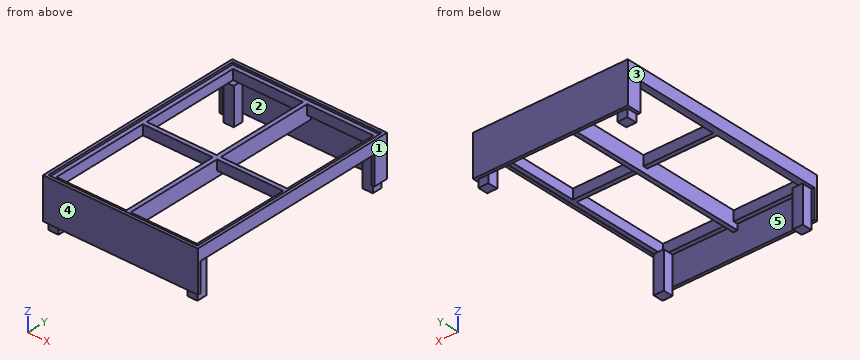
```python
from build123d import *

# Parameters (mm, degrees)
F0_W      = 1371.6
F0_H      = 1905
F0_W_2    = 1320.8
F0_H_2    = 1854.2
F1_DEPTH  = 365.125
F2_W      = 38.1
F2_H      = 139.7
F3_DEPTH  = 1854.2
F4_W      = 1854.2
F4_H      = 88.9
F5_DEPTH  = 38.1
F6_W      = 1854.2
F6_H      = 88.9
F7_DEPTH  = 38.1
F8_W      = 1752.6
F8_H      = 254
F9_DEPTH  = 1371.601
F10_DEPTH = 1752.6
F11_W     = 38.1
F11_H     = 88.9
F12_DEPTH = 1270
F13_W     = 38.1
F13_H     = 88.9
F14_DEPTH = 1270
F15_W     = 38.1
F15_H     = 88.9
F16_DEPTH = 1270
F17_W     = 88.9
F17_H     = 88.9
F18_DEPTH = 327.025
F19_W     = 88.9
F19_H     = 88.9
F20_DEPTH = 327.025
F21_W     = 88.9
F21_H     = 88.9
F22_DEPTH = 327.025
F23_W     = 88.9
F23_H     = 88.9
F24_DEPTH = 327.025


with BuildPart() as f1:
    # F0 (on Top) → F1 (new body)
    with BuildSketch(Plane.XY):
        Rectangle(F0_W, F0_H)
        Rectangle(F0_W_2, F0_H_2, mode=Mode.SUBTRACT)
    extrude(amount=F1_DEPTH)

    # F2 (on face) → F3 (join, through all)
    with BuildSketch(Plane.XZ.offset(-927.1)):
        with Locations((15.875, 276.225)):
            Rectangle(F2_W, F2_H)
    extrude(amount=F3_DEPTH)

    # F4 (on face) → F5 (join)
    with BuildSketch(Plane.YZ.offset(-660.4)):
        with Locations((0, 301.625)):
            Rectangle(F4_W, F4_H)
    extrude(amount=F5_DEPTH)

    # F6 (on face) → F7 (join)
    with BuildSketch(Plane(origin=(660.4, 0, 0), x_dir=(0, -1, 0), z_dir=(-1, 0, 0))):
        with Locations((0, 301.625)):
            Rectangle(F6_W, F6_H)
    extrude(amount=F7_DEPTH)

    # F8 (on face) → F9 (cut, through all)
    with BuildSketch(Plane.YZ.offset(685.8)):
        with Locations((-50.8, 127)):
            Rectangle(F8_W, F8_H)
    extrude(amount=-F9_DEPTH, mode=Mode.SUBTRACT)

    # F10 (add, through all): a face of the model
    f10_faces = [f1.faces().sort_by_distance(p)[0] for p in [
        (15.875, 825.5, 230.1875),
    ]]
    extrude(f10_faces, amount=F10_DEPTH)

    # F11 (on face) → F12 (join)
    with BuildSketch(Plane.YZ.offset(-622.3)):
        with Locations((908.05, 301.625)):
            Rectangle(F11_W, F11_H)
    extrude(amount=F12_DEPTH)

    # F13 (on face) → F14 (join)
    with BuildSketch(Plane.YZ.offset(-622.3)):
        with Locations((-908.05, 301.625)):
            Rectangle(F13_W, F13_H)
    extrude(amount=F14_DEPTH)

    # F15 (on face) → F16 (join)
    with BuildSketch(Plane.YZ.offset(-622.3)):
        with Locations((0, 301.625)):
            Rectangle(F15_W, F15_H)
    extrude(amount=F16_DEPTH)

    # F17 (on face) → F18 (join)
    with BuildSketch(Plane(origin=(0, 0, 257.175), x_dir=(1, 0, 0), z_dir=(0, 0, -1))):
        with Locations((-615.95, 882.65)):
            Rectangle(F17_W, F17_H)
    extrude(amount=F18_DEPTH)

    # F19 (on face) → F20 (join)
    with BuildSketch(Plane(origin=(0, 0, 257.175), x_dir=(1, 0, 0), z_dir=(0, 0, -1))):
        with Locations((615.95, 882.65)):
            Rectangle(F19_W, F19_H)
    extrude(amount=F20_DEPTH)

    # F21 (on face) → F22 (join)
    with BuildSketch(Plane(origin=(0, 0, 257.175), x_dir=(1, 0, 0), z_dir=(0, 0, -1))):
        with Locations((-615.95, -882.65)):
            Rectangle(F21_W, F21_H)
    extrude(amount=F22_DEPTH)

    # F23 (on face) → F24 (join)
    with BuildSketch(Plane(origin=(0, 0, 257.175), x_dir=(1, 0, 0), z_dir=(0, 0, -1))):
        with Locations((615.95, -882.65)):
            Rectangle(F23_W, F23_H)
    extrude(amount=F24_DEPTH)


solid = f1.part
```
Read the model definition and answer for the solid it produces. Units are mm, in the model's axes. Face numbers are marked on the shaded views. A direction names the side the tool comes from. Coordinates: 2 decimals unless noted, no trailing zeros. Order: outer loops, then holes, each group sorted by start corner. A loop starts at its lowest first (then second) coordinate and runs counter-clockwise, first axis right, second up. Notation, with made-up numbers: (-38, 52) - (13, 52) arc R18 cw to (13, 87) - close; hole circle Ø6 at (59, 25.5). An arc over 180 degrees is marked (long way). Answer as a JSON object with one key per item and string values. Group by question number.
Item 1: Consider probe 1 along Y at (x, z) = (-561.5, 299); probe 2 along X at (y, z) = (-777, 334) (3 decimals); probe 3 along Y at (x, z) = (-570.5, 108.5). Determine where each line is inside the solid, lowest interval first. Write a range as from..to.
Item 2: Section C-C (y = 122) is taken. Give the vertices of the cut face in (x, z) (3 decimals).
Item 3: Section B-B (x = 305.5) is taken. Give the vertices of the cut face in (y, z) (3 decimals).
Item 4: A flat-ended cylindrical pin translates along its axis: P1, Ø4, axis at x = 538.5, y = 9, coming from the +Z side (3 decimals). Find the tip coordinate at first contact, or state that the pin passes through.
Item 5: Section D-D (z = 290) is taken. Give the vertices of the cut face in (x, y) (3 decimals).
Item 6: Section A-A (z = 149) is taken. Give the vertices of the cut face in (x, y).
Item 7: A tool of negligible diameter and unlimited length cuts with its end or side. For the marked faces 1 and 2, from which of +Z, -Z, +X, -X, +Y, -Y can it reach the whole face along a straight path? Write none if from no direction.
Item 8: The mould has two halves that part along Y. Classify the marked faces 3, 4 and 5: +Y half, -Y half, draft (parallel to the pull), parting line (faces both ways), or undercut.
Results are:
{
 "1": {"probe 1": "y = -952.5..-889, -19.05..19.05, 889..952.5", "probe 2": "x = -685.8..-622.3, -3.175..34.925, 622.3..685.8", "probe 3": "y = -952.5..-927.1, 927.1..952.5"},
 "2": {"outline": "(-685.8, 254) - (-660.4, 254) - (-660.4, 257.175) - (-622.3, 257.175) - (-622.3, 346.075) - (-660.4, 346.075) - (-660.4, 365.125) - (-685.8, 365.125) - close; (-3.175, 206.375) - (34.925, 206.375) - (34.925, 346.075) - (-3.175, 346.075) - close; (622.3, 257.175) - (660.4, 257.175) - (660.4, 254) - (685.8, 254) - (685.8, 365.125) - (660.4, 365.125) - (660.4, 346.075) - (622.3, 346.075) - close"},
 "3": {"outline": "(-952.5, 0) - (-927.1, 0) - (-927.1, 257.175) - (-889, 257.175) - (-889, 346.075) - (-927.1, 346.075) - (-927.1, 365.125) - (-952.5, 365.125) - close; (-19.05, 257.175) - (19.05, 257.175) - (19.05, 346.075) - (-19.05, 346.075) - close; (889, 257.175) - (927.1, 257.175) - (927.1, 0) - (952.5, 0) - (952.5, 365.125) - (927.1, 365.125) - (927.1, 346.075) - (889, 346.075) - close"},
 "4": {"P1": "stops at z = 346.075"},
 "5": {"outline": "(-685.8, -952.5) - (685.8, -952.5) - (685.8, 952.5) - (-685.8, 952.5) - close; hole (-622.3, -889) - (-3.175, -889) - (-3.175, -19.05) - (-622.3, -19.05) - close; hole (-622.3, 19.05) - (-3.175, 19.05) - (-3.175, 889) - (-622.3, 889) - close; hole (34.925, -889) - (622.3, -889) - (622.3, -19.05) - (34.925, -19.05) - close; hole (34.925, 19.05) - (622.3, 19.05) - (622.3, 889) - (34.925, 889) - close"},
 "6": {"outline": "(-685.8, -952.5) - (685.8, -952.5) - (685.8, -927.1) - (660.4, -927.1) - (660.4, -838.2) - (571.5, -838.2) - (571.5, -927.1) - (-571.5, -927.1) - (-571.5, -838.2) - (-660.4, -838.2) - (-660.4, -927.1) - (-685.8, -927.1) - close; (-685.8, 825.5) - (-660.4, 825.5) - (-660.4, 838.2) - (-571.5, 838.2) - (-571.5, 927.1) - (571.5, 927.1) - (571.5, 838.2) - (660.4, 838.2) - (660.4, 825.5) - (685.8, 825.5) - (685.8, 952.5) - (-685.8, 952.5) - close"},
 "7": {"face 1": "+Z, -Z, +X, +Y, -Y", "face 2": "-Z"},
 "8": {"face 3": "draft", "face 4": "-Y half", "face 5": "undercut"}
}
